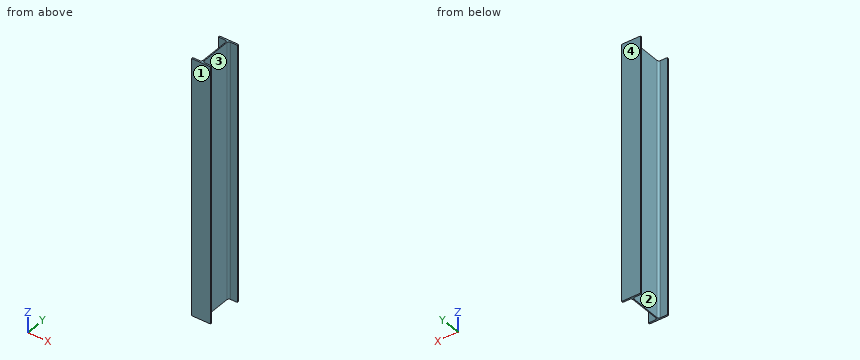
Autodesk Inventor part; units mm, degrees
ref_plane "Start plane" through (0, 0, 0) normal (0, 0, 1) x (1, 0, 0)
ref_plane "End plane" through (0, 0, 1500) normal (0, 0, 1) x (1, 0, 0)
ref_plane "YZ Plane" through (0, 0, 0) normal (1, 0, 0) x (0, 1, 0)
ref_plane "Start plane" through (0, 0, 0) normal (0, 0, 1) x (1, 0, 0)
ref_plane "End plane" through (0, 0, 1500) normal (0, 0, 1) x (1, 0, 0)
sketch "Sketch2" plane through (0, 0, 0) normal (0, 0, 1) x (1, 0, 0)
  line L0 (-55, 100.8) -> (-14.95, 100.8)
  line L1 (-55, 110) -> (-55, 100.8)
  line L2 (55, 110) -> (-55, 110)
  line L3 (55, 100.8) -> (55, 110)
  line L4 (14.95, 100.8) -> (55, 100.8)
  line L5 (2.95, -88.8) -> (2.95, 88.8)
  line L6 (55, -100.8) -> (14.95, -100.8)
  line L7 (55, -110) -> (55, -100.8)
  line L8 (-55, -100.8) -> (-55, -110)
  line L9 (-14.95, -100.8) -> (-55, -100.8)
  line L10 (-2.95, 88.8) -> (-2.95, -88.8)
  line L11 (0, -252) -> (0, 252) construction
  line L12 (-2.95, -100.8) -> (2.95, -100.8) construction
  arc A0 (-14.95, -100.8) -> (-2.95, -88.8) centre (-14.95, -88.8) ccw
  arc A1 (-2.95, 88.8) -> (-14.95, 100.8) centre (-14.95, 88.8) ccw
  arc A2 (14.95, 100.8) -> (2.95, 88.8) centre (14.95, 88.8) ccw
  arc A3 (2.95, -88.8) -> (14.95, -100.8) centre (14.95, -88.8) ccw
  line L13 (-119, 0) -> (119, 0) construction
  line L14 (-55, -110) -> (55, -110)
  point P0 (-2.95, 100.8)
  point P1 (2.95, 100.8)
  point P2 (0, 0)
  point P3 (0, -100.8)
  point P4 (0, 0)
  dimension "d1" = 220
  dimension "d3" = 9.2
  dimension "d5" = 5.9
  dimension "d7" = 110
  dimension "d13" = 12
  dimension "d14" = 110
  dimension "d15" = 55
extrude "Body" add sketch "Sketch2" along normal up to surface (1500 mm away) from surface at 0
sketch "Sketch3" plane through (0, 0, 0) normal (0, 0, 1) x (1, 0, 0)
  line L0 (0, 0) -> (10, 0)
ref_plane "Work Plane3" through (0, 0, 0) normal (0, -1, 0) x (1, 0, 0)
sketch "Sketch4" plane through (0, 0, 0) normal (0, -1, 0) x (1, 0, 0)
  line L0 (-2, 0) -> (12, 0)
  line L1 (-2, 1500) -> (12, 1500)
  dimension "d19" = 1500
equation "\"d1\" = ParH"
equation "\"d3\" = t2"
equation "\"d7\" = b"
equation "\"d13\" = R1"
equation "\"d14\" = 0.5 * d1"
equation "\"d15\" = 0.5 * d7"
equation "\"d8\" = G_L"
equation "\"b\" = 110"
equation "\"ParH\" = 220"
equation "\"R1\" = 12"
equation "\"G_L\" = d19"
equation "\"t1\" = 5.9"
equation "\"t2\" = 9.2"
equation "\"G_OFFSET_START\" = 0"
equation "\"G_OFFSET_END\" = 0"
properties part number "DIN 1025 - IPE 220-1500" material "Steel, Mild"
Part model, mm, in its own coordinate system. Face numbers are marked on the shaded views. Coordinates: 2 decimals unless noted, no trailing zeros. Order: outer loops, then holes, each group sorted by start corner. A loop starts at its lowest first (then second) coordinate and runs counter-clockwise, first axis right, second up. Notation, with made-up numbers: (82, 31.5) - (128, 31.5) arc R13 cw to (128, 53.5) - close; hole circle Ø6 at (-28, 0). An arc over 180 degrees is marked (long way). Return JSON: item names as keys, results as strings. Group by question number.
Item 1: Drill centre lines: probe 1 along Y at (x, z) = (37, 342); probe 2 along X at (y, z) = (13, 125); probe 3 along Y at (x, z) = (-5.5, 1396). Where is each one in solid material? Low to high. Write a range as from..to.
Item 2: Pin check, flat tip, straight feed: pin 1 (12 mm diameter, centred on y = -56, z = 930.5, fed in from +X). Stop position of the tip, or through.
Item 3: Pull direction Y, two halves, no side cores. Call the marked faces 1, 2, 3 and 4: pulls with the +Y half, pulls with the -Y half, needs draft (parallel to the pull), parting line crosses it, or undercut.
Item 4: Cut at B-B (z = 1134). List the corners of the cut face in (x, y).
Item 5: Cut at C-C (y = -14). List the corners of the cut face in (x, z), plus the area to 3 significant figures.
Item 6: Cut at A-A (x = 29). List the corners of the cut face in (y, z), plus the area to 3 significant figures.
Check values:
{
 "1": {"probe 1": "y = -110..-100.8, 100.8..110", "probe 2": "x = -2.95..2.95", "probe 3": "y = -110..-96.2, 96.2..110"},
 "2": {"pin 1": "stops at x = 2.95"},
 "3": {"face 1": "pulls with the -Y half", "face 2": "undercut", "face 3": "undercut", "face 4": "pulls with the +Y half"},
 "4": {"outline": "(-55, -110) - (55, -110) - (55, -100.8) - (14.95, -100.8) arc R12 cw to (2.95, -88.8) - (2.95, 88.8) arc R12 cw to (14.95, 100.8) - (55, 100.8) - (55, 110) - (-55, 110) - (-55, 100.8) - (-14.95, 100.8) arc R12 cw to (-2.95, 88.8) - (-2.95, -88.8) arc R12 cw to (-14.95, -100.8) - (-55, -100.8) - close"},
 "5": {"outline": "(-2.95, 0) - (2.95, 0) - (2.95, 1500) - (-2.95, 1500) - close", "area": "8,850 mm2"},
 "6": {"outline": "(-110, 0) - (-100.8, 0) - (-100.8, 1500) - (-110, 1500) - close; (100.8, 0) - (110, 0) - (110, 1500) - (100.8, 1500) - close", "area": "27,600 mm2"}
}
